from build123d import *

# Parameters (mm, degrees)
F0_R        = 3
F1_DEPTH    = 10
F2_R        = 5
F3_R        = 4.99999
F4_T1_DEPTH = 10
F4_T3_DEPTH = 15.1433659759
F4_T5_DEPTH = 12.2571417204


# Not quite as in the source:
# - a fillet or chamfer that OpenCascade refuses, or shapes differently, is made with other operations: its cross-section is extruded or revolved along the edge and cut away or added
# - a fillet or chamfer is up to 0.001 mm smaller than in the source, because OpenCascade refuses the exact size


with BuildPart() as f1:
    # F0 (on Top) → F1 (new body)
    with BuildSketch(Plane.XY):
        with BuildLine():
            Line((18, 18), (0, 0))
            Line((0, 0), (-11, 11))
            ThreePointArc((-11, 11), (-12.8659446975, 12.2241130817), (-12.4367385267, 14.4140867148))
            Line((-12.4367385267, 14.4140867148), (-11, 15.8508252416))
            Line((-11, 15.8508252416), (-11, 21.9997463049))
            Line((-11, 21.9997463049), (-23, 21.9997463049))
            Line((-23, 21.9997463049), (-23, 1.9289321881))
            Line((-23, 1.9289321881), (-6.5, -14.5710678119))
            Line((-6.5, -14.5710678119), (-6.5, -94.5710678119))
            Line((-6.5, -94.5710678119), (6.5, -94.5710678119))
            Line((6.5, -94.5710678119), (6.5, -14.5710678119))
            Line((6.5, -14.5710678119), (25.0710678119, 4))
            Line((25.0710678119, 4), (25.0710678119, 18))
            Line((25.0710678119, 18), (18, 18))
        make_face()
        with Locations((20.0710678119, 13)):
            Circle(F0_R, mode=Mode.SUBTRACT)
    extrude(amount=F1_DEPTH)

    # F2
    f2_edges = [f1.edges().sort_by_distance(p)[0] for p in [
        (18, 18, 5),
    ]]
    fillet(f2_edges, radius=F2_R)

    # F3 (radius 5 in the source; OpenCascade refuses exactly that, so slightly less here)
    f3_edges = [f1.edges().sort_by_distance(p)[0] for p in [
        (25.071068, 18, 5),
    ]]
    fillet(f3_edges, radius=F3_R)

    # F4: chamfer of 1 on 5 edges, made by hand

    # F4_s2 → F4_t1 (join)
    with BuildSketch(Plane.XY):
        Polygon((-6.5, -14.9852813742), (-6.7928932188, -14.2781745931), (-6.5, -14.5710678119), align=None)
        Polygon((6.7928932188, -14.2781745931), (6.5, -14.9852813742), (6.5, -14.5710678119), align=None)
    extrude(amount=F4_T1_DEPTH)

    # F4_s4 → F4_t3 (cut)
    with BuildSketch(Plane.XY.offset(-2.571682988)):
        Polygon((-11, 20.9997463049), (-12, 21.9997463049), (-11, 21.9997463049), align=None)
        Polygon((-22, 21.9997463049), (-23, 20.9997463049), (-23, 21.9997463049), align=None)
    extrude(amount=F4_T3_DEPTH, mode=Mode.SUBTRACT)

    # F4_s6 → F4_t5 (cut)
    with BuildSketch(Plane.XY.offset(-1.1285708602)):
        Polygon((-22.7071067812, 1.6360389693), (-23, 2.3431457505), (-23, 1.9289321881), align=None)
    extrude(amount=F4_T5_DEPTH, mode=Mode.SUBTRACT)


solid = f1.part
The listing builds one solid part. Answer for the finished solid, in the listing's coordinates (mm). A direction names the side the tool comes from. Round coordinates to 2 decimals unless told otherwise and drop trailing zeros. Order: outer loops, then holes, each group sorted by start corner. A loop starts at its lowest first (then second) coordinate and runs counter-clockwise, first axis right, second up. Notation, with made-up numbers: M -39,82.5 L -34,82.5 A11 cw -34,102.5 Z; hole C 5.25,29.5 d1. An arc over 180 degrees is marked long. Answer in a Markdown table with one row per item. Add a question column.
1) The part is cut by section C-C on y = -47. Determine the outline of the cut face in (x, z).
2) Consider line 1 along X through (y, z) = (-74.5, 2); line 2 along Y through (x, z) = (-8, 7.75); line 3 along Y through (x, z) = (-18, 9). Determine where each line is inside the solid, lowest interval first. Write a range as from..to.
3) The part is cut by section A-A on y = 8.5. Determine the outline of the cut face in (x, z).
4) Flat-ended cylindrical pins translate along their axes: pin 1 Ø6 at (x, z) = (10.5, 1.5) entering from +Y; pin 2 Ø2 at (x, z) = (2, 4) entering from +Y; pin 3 Ø12 at (x, y) = (8, -12) entering from -Z; pin 4 Ø6 at (y, z) = (-8, 4.5) entering from +X. Find the tip coordinate at first contact, or state that the pin passes through.
5) The part is cut by section D-D on x = 12. Determine the outline of the cut face in (y, z).
6) Determine the mould class of faces 6 (the face through (8, 8, 5)), 7 (the face through (18.13, 17.61, 5.07)), 8 (the face through (-1, -27, 0)), 9 (the face through (25.071, 8, 5)) for opening direction X: pulls with the +X half, pulls with the -X half, needs draft (parallel to the pull), parting line crosses it, or undercut.
7) Which of the six approach directions +Z, -Z, +X, -X, +Y, -Y give full straight-line access (tool end or side, diameter ignored) to faces 1 (the face through (6.5, -55, 5)), 2 (the face through (-11, 18, 5)), 3 (the face through (-12.85, 12.19, 4.93)), 4 (the face through (-6.5, -54, 5)), 5 (the face through (23.57, 16.57, 5.07))?
Findings below:
| question | item | result |
|---|---|---|
| 1 | outline | M -6.5,0 L 6.5,0 L 6.5,10 L -6.5,10 Z |
| 2 | line 1 | x = -6.5..6.5 |
| 2 | line 2 | y = -13.07..8 |
| 2 | line 3 | y = -3.07..22 |
| 3 | outline | M -23,0 L -8.5,0 L -8.5,10 L -23,10 Z; M 8.5,0 L 25.07,0 L 25.07,10 L 8.5,10 Z |
| 4 | pin 1 | stops at y = 13.5 |
| 4 | pin 2 | stops at y = 3 |
| 4 | pin 3 | stops at z = 0 |
| 4 | pin 4 | stops at x = 16.07 |
| 5 | outline | M -9.07,0 L 12,0 L 12,10 L -9.07,10 Z |
| 6 | face 6 | undercut |
| 6 | face 7 | undercut |
| 6 | face 8 | needs draft |
| 6 | face 9 | pulls with the +X half |
| 7 | face 1 | +Z, -Z, +X, -Y |
| 7 | face 2 | +Z, -Z, +Y |
| 7 | face 3 | +Z, -Z |
| 7 | face 4 | +Z, -Z, -X, -Y |
| 7 | face 5 | +Z, -Z, +X, +Y |
